```python
from build123d import *

# Parameters (mm, degrees)
SKETCH1_W           = 89.973098965
SKETCH1_H           = 90.646237782
BOSS_EXTRUDE1_DEPTH = 3.175


with BuildPart() as part:
    # Sketch1 → Boss-Extrude1 (new body)
    with BuildSketch(Plane.XY):
        Polygon((311.775650515, 151.416855126), (311.775650515, 135.470394989), (308.79500376, 135.470394989), (308.79500376, 118.65457955), (313.017586662, 118.65457955), (313.017586662, 116.543288099), (313.017586662, 114.431996648), (308.79500376, 114.431996648), (308.79500376, 97.616181208), (311.775650515, 97.616181208), (311.775650515, 59.761967427), (308.79500376, 59.761967427), (308.79500376, 42.946151987), (313.017586662, 42.946151987), (313.017586662, 40.834860536), (313.017586662, 38.723569085), (308.79500376, 38.723569085), (308.79500376, 21.907753645), (311.775650515, 21.907753645), (311.775650515, 5.961293509), (327.722110651, 5.961293509), (327.722110651, 2.980646754), (344.53792609, 2.980646754), (344.53792609, 7.203229657), (346.649217542, 7.203229657), (348.760508993, 7.203229657), (348.760508993, 2.980646754), (365.576324432, 2.980646754), (365.576324432, 5.961293509), (403.430538214, 5.961293509), (403.430538214, 2.980646754), (420.246353653, 2.980646754), (420.246353653, 7.203229657), (422.357645104, 7.203229657), (424.468936555, 7.203229657), (424.468936555, 2.980646754), (441.284751995, 2.980646754), (441.284751995, 5.961293509), (457.231212131, 5.961293509), (457.231212131, 21.907753645), (460.211858886, 21.907753645), (460.211858886, 38.723569085), (455.989275984, 38.723569085), (455.989275984, 40.834860536), (455.989275984, 42.946151987), (460.211858886, 42.946151987), (460.211858886, 59.761967427), (457.231212131, 59.761967427), (457.231212131, 97.616181208), (460.211858886, 97.616181208), (460.211858886, 114.431996648), (455.989275984, 114.431996648), (455.989275984, 116.543288099), (455.989275984, 118.65457955), (460.211858886, 118.65457955), (460.211858886, 135.470394989), (457.231212131, 135.470394989), (457.231212131, 151.416855126), (441.284751995, 151.416855126), (441.284751995, 154.39750188), (424.468936555, 154.39750188), (424.468936555, 150.174918978), (422.357645104, 150.174918978), (420.246353653, 150.174918978), (420.246353653, 154.39750188), (403.430538214, 154.39750188), (403.430538214, 151.416855126), (365.576324432, 151.416855126), (365.576324432, 154.39750188), (348.760508993, 154.39750188), (348.760508993, 150.174918978), (346.649217542, 150.174918978), (344.53792609, 150.174918978), (344.53792609, 154.39750188), (327.722110651, 154.39750188), (327.722110651, 151.416855126), align=None)
        with Locations((384.387424227, 78.399039157)):
            Rectangle(SKETCH1_W, SKETCH1_H, mode=Mode.SUBTRACT)
    extrude(amount=BOSS_EXTRUDE1_DEPTH)


solid = part.part
```
Part model, mm, in its own coordinate system. Round coordinates to 2 decimals unless told otherwise and drop trailing zeros. Write each loop counter-clockwise with the first axis right and the second up, starting at its lowest first coordinate (ties: lowest second). Pieces come first, ordered by that corner, then holes. Notation, with made-up numbers: M 17,14 L 52,14 A17 ccw 52,47 Z; hole C -25,2.5 d8. An arc over 180 degrees is marked long. One line per question, with ' | ' between items.
(1) Saw through at C-C on x = 451.5. Write the cut outline in (y, z) (3 decimals), then the cut area to 3 significant figures.
Answer key:
outline: M 5.961,0 L 151.417,0 L 151.417,3.175 L 5.961,3.175 Z | area: 462 mm^2
(2) Pin check, flat tips, straight feed: pin 1 (1 mm diameter, centred on x = 311.5, z = 1.5, fed in from -Y); pin 2 (1.6 mm diameter, centred on y = 151.5, z = 1.5, fed in from +X); pin 3 (1 mm diameter, centred on y = 151.5, z = 2, fed in from -X). Stop position of each tip, or through.
Answer key:
pin 1: stops at y = 5.96 | pin 2: stops at x = 457.23 | pin 3: stops at x = 311.78
(3) Saw through at B-B on y = 57. Write the cut outline in (x, z) (3 decimals).
Answer key:
outline: M 308.795,0 L 339.401,0 L 339.401,3.175 L 308.795,3.175 Z; M 429.374,0 L 460.212,0 L 460.212,3.175 L 429.374,3.175 Z
(4) Probe line 1 along X through (y, z) = (88.5, 2.95); line 2 along X through (y, z) = (38, 2.3) (3 decimals); line 3 along Y through (x, z) = (376.5, 0.9). List the from-to ranges inside material, lowest first.
Answer key:
line 1: x = 311.78 to 339.4, 429.37 to 457.23 | line 2: x = 308.795 to 339.401, 429.374 to 460.212 | line 3: y = 5.96 to 33.08, 123.72 to 151.42
(5) Saw through at A-A on y = 85. Write the cut outline in (x, z) (3 decimals).
Answer key:
outline: M 311.776,0 L 339.401,0 L 339.401,3.175 L 311.776,3.175 Z; M 429.374,0 L 457.231,0 L 457.231,3.175 L 429.374,3.175 Z
